```python
from build123d import *

# Parameters (mm, degrees)
F0_R     = 12.7
F1_DEPTH = 57.15
F2_R     = 4.7625
F3_DEPTH = 44.45
F4_R     = 2.54
F5_SIZE  = 0.3


with BuildPart() as f1:
    # F0 (on Top) → F1 (new body)
    with BuildSketch(Plane.XY):
        Circle(F0_R)
    extrude(amount=F1_DEPTH)

    # F2 (on face) → F3 (cut)
    with BuildSketch(Plane.XY.offset(57.15)):
        Circle(F2_R)
    extrude(amount=-F3_DEPTH, mode=Mode.SUBTRACT)

    # F4
    f4_edges = [f1.edges().sort_by_distance(p)[0] for p in [
        (-12.7, 0, 0),
        (-12.7, 0, 57.15),
    ]]
    fillet(f4_edges, radius=F4_R)

    # F5
    f5_edges = [f1.edges().sort_by_distance(p)[0] for p in [
        (-4.7625, 0, 12.7),
        (-10.16, 0, 57.15),
        (-4.7625, 0, 57.15),
    ]]
    chamfer(f5_edges, length=F5_SIZE)


solid = f1.part
```
Geometry check sheet. Reference: the model listing, model coordinates, mm. Give positions to 0.01 mm unless a question says otherwise; leave off trailing zeros. Order: outer loops, then holes, each group sorted by start corner. A loop starts at its lowest first (then second) coordinate and runs counter-clockwise, first axis right, second up. Notation, with made-up numbers: (69, 24) - (117, 24) arc R23 ccw to (117, 32) - close; hole circle Ø2 at (61, 62). An arc over 180 degrees is marked (long way). Answer in a Markdown table with one row per item. Add a question column.
Q1. Cross-section at A-A, the plane y = 0. Enter the section's corners in (x, z).
Q2. Material ranges on probe 1 along Y at (x, z) = (0, 44); probe 2 along Z at (x, y) = (0, -3); probe 3 along X at (y, z) = (0.75, 43), recorded low to high. Write a range as from..to.
Q3. Cross-section at B-B, the plane z = 40. Enter the section's corners in (x, y) (1 decimal).
Q4. Gauge pin test, flat ends, axial feed: pin 1 (1 mm diameter, centred on y = 7, z = 23.5, fed in from -X); pin 2 (2 mm diameter, centred on x = 6, z = 14, fed in from -Y); pin 3 (8 mm diameter, centred on y = -9, z = 6.5, fed in from +X). Record the tip position at first contact, or that the pin passes through.
Q5. Cross-section at D-D, the plane z = 6. Enter the section's corners in (x, y), then the cut area to 3 significant figures.
Q6. Mould release check, pull along X, two halves, no side actions. Record for faces 1 (the cylindrical face through (-2.75, -12.4, 28.21)), 2 (the flat face through (0, 0, 0)), 3 (the flat face through (0, 0, 12.7)), 4 (the cylindrical face through (-3.78, -2.9, 35.23)): pulls with the +X half, pulls with the -X half, needs draft (parallel to the pull), parting line crosses it, or undercut.
Check values:
| question | item | result |
|---|---|---|
| 1 | outline | (-12.7, 2.54) arc R2.54 ccw to (-10.16, 0) - (10.16, 0) arc R2.54 ccw to (12.7, 2.54) - (12.7, 54.61) arc R2.54 ccw to (10.16, 57.15) - (5.06, 57.15) - (4.76, 56.85) - (4.76, 13) - (4.46, 12.7) - (-4.46, 12.7) - (-4.76, 13) - (-4.76, 56.85) - (-5.06, 57.15) - (-10.16, 57.15) arc R2.54 ccw to (-12.7, 54.61) - close |
| 2 | probe 1 | y = -12.7..-4.76, 4.76..12.7 |
| 2 | probe 2 | z = 0..12.7 |
| 2 | probe 3 | x = -12.68..-4.7, 4.7..12.68 |
| 3 | outline | circle Ø25.4 at (0, 0); hole circle Ø9.5 at (0, 0) |
| 4 | pin 1 | stops at x = -10.91 |
| 4 | pin 2 | stops at y = -11.67 |
| 4 | pin 3 | stops at x = 11.67 |
| 5 | outline | circle Ø25.4 at (0, 0) |
| 5 | area | 507 mm^2 |
| 6 | face 1 | parting line crosses it |
| 6 | face 2 | needs draft |
| 6 | face 3 | undercut |
| 6 | face 4 | undercut |
